Study the drawing (mm; zero at the part's minimum x, y, z) and answer. Give positions to 0.01 mm unless a question says otherwise; leave off trailing zeros. Order: outer loops, then holes, each group sorted by start corner. A loop starts at its lowest first (then second) coordinate and runs counter-clockwise, first axis right, second up.
Item 1: A cutting plane is placed at A-A (x = 1302.5). Write down the section's boundary in (y, z) (1 decimal).
Item 2: A cutting plane is placed at B-B (y = 12.5). Write down the section's boundary in (x, z).
Item 3: Given pin 1 Ø3 at (y, z) = (5, 781.5) entering from -X; pin 2 Ø12 at (y, z) = (8.5, 1136.5) entering from +X; pin 3 Ø5 at (y, z) = (21.5, 975) entering from -X, each flat-ended and moving along its own axis, determine where each tip first touches the part or whether it passes through.
Item 4: A cutting plane is placed at D-D (x = 432). Write down the section's boundary in (y, z) (1 decimal).
Item 5: A cutting plane is placed at C-C (z = 923). Write down the section's boundary in (x, y), plus the area to 3 significant figures.
Item 6: Find the intervals of material crossed by line 1 along Z through (x, y) = (1577, 8.25); line 2 along Z through (x, y) = (316.5, 18); line 3 along Z through (x, y) = (1016, 6), in increasing order.
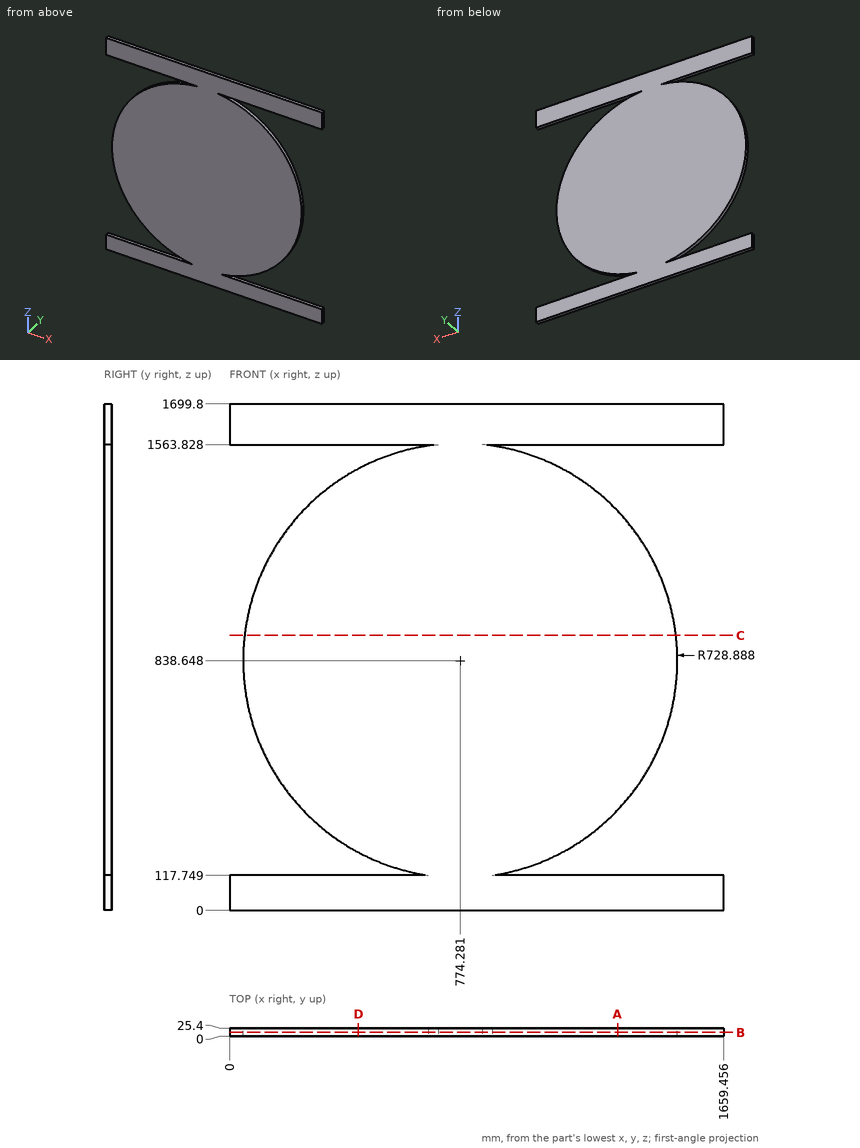
Response values:
1. outline: (0, 0) - (25.4, 0) - (25.4, 117.7) - (0, 117.7) - close; (0, 336.4) - (25.4, 336.4) - (25.4, 1340.9) - (0, 1340.9) - close; (0, 1563.8) - (25.4, 1563.8) - (25.4, 1699.8) - (0, 1699.8) - close
2. outline: (0, 0) - (1659.46, 0) - (1659.46, 117.75) - (881.9, 117.75) arc R728.89 ccw to (847.71, 1563.83) - (1659.46, 1563.83) - (1659.46, 1699.8) - (0, 1699.8) - (0, 1563.83) - (700.85, 1563.83) arc R728.89 ccw to (666.66, 117.75) - (0, 117.75) - close
3. pin 1: stops at x = 47.52
3. pin 2: stops at x = 1442.19
3. pin 3: stops at x = 57.79
4. outline: (0, 0) - (25.4, 0) - (25.4, 117.7) - (0, 117.7) - close; (0, 195.1) - (25.4, 195.1) - (25.4, 1482.2) - (0, 1482.2) - close; (0, 1563.8) - (25.4, 1563.8) - (25.4, 1699.8) - (0, 1699.8) - close
5. outline: (50.29, 0) - (1498.27, 0) - (1498.27, 25.4) - (50.29, 25.4) - close
5. area: 36,800 mm2
6. line 1: z = 0 to 117.75, 1563.83 to 1699.8
6. line 2: z = 0 to 117.75, 271.45 to 1405.85, 1563.83 to 1699.8
6. line 3: z = 0 to 117.75, 151.01 to 1526.29, 1563.83 to 1699.8
